Could you check a few things on this model? Use its own coordinates, in mm. A direction names the side the tool comes from. Round coordinates to 2 decimals unless told otherwise and drop trailing zeros. Order: outer loops, then holes, each group sorted by start corner. A loop starts at its lowest first (then second) coordinate and runs counter-clockwise, first axis right, second up. Notation, with made-up numbers: (40.25, 11.5) - (69.25, 11.5) arc R32 ccw to (69.25, 42.5) - close; hole circle Ø2 at (-30, 18.25). An arc over 180 degrees is marked (long way). Use one line per item in the form item = value.
from build123d import *

# Parameters (mm, degrees)
F0_R     = 100
F1_DEPTH = 3
F2_R     = 80
F3_DEPTH = 15
F4_R     = 77
F5_DEPTH = 18.001
F6_R     = 2.1
F6_R_2   = 2
F6_R_3   = 1
F7_DEPTH = 3.001


with BuildPart() as f1:
    # F0 (on Front) → F1 (new body)
    with BuildSketch(Plane.XZ):
        Circle(F0_R)
    extrude(amount=F1_DEPTH)

    # F2 (on face) → F3 (join)
    with BuildSketch(Plane.XZ.offset(3)):
        Circle(F2_R)
    extrude(amount=F3_DEPTH)

    # F4 (on face) → F5 (cut, through all)
    with BuildSketch(Plane.XZ.offset(18)):
        Circle(F4_R)
    extrude(amount=-F5_DEPTH, mode=Mode.SUBTRACT)

    # F6 (on face) → F7 (cut, through all)
    with BuildSketch(Plane.XZ.offset(3)):
        with Locations((80.622577, 40)):
            Circle(F6_R)
        with Locations((-80.622577, 40)):
            Circle(F6_R_2)
        with Locations((-80.622577, -40)):
            Circle(F6_R_2)
        with Locations((80.622577, -40)):
            Circle(F6_R_2)
        with Locations((80.770344, 0)):
            Circle(F6_R_3)
    extrude(amount=-F7_DEPTH, mode=Mode.SUBTRACT)


solid = f1.part
Item 1: Imagine slicing it at A-A on x = 0. Please give me the cut outline in (y, z).
Found:
outline = (-18, -80) - (-3, -80) - (-3, -100) - (0, -100) - (0, -77) - (-18, -77) - close; (-18, 77) - (0, 77) - (0, 100) - (-3, 100) - (-3, 80) - (-18, 80) - close
Item 2: Will these pins go through, and if not, where does the flat tip stop? P1, Ø3, axis at x = 14.5, y = -11, coming from the +Z side; P2, Ø1.5, axis at x = 26, y = -15.5, coming from the -Z side; P3, Ø4.5, axis at x = -80.62, z = 40, coming from the -Y side.
Found:
P1 = 78.94
P2 = -75.91
P3 = -3
Item 3: Imagine slicing it at D-D on x = -86. Please give me the cut outline in (y, z).
Found:
outline = (-3, -51.03) - (0, -51.03) - (0, 51.03) - (-3, 51.03) - close
Item 4: Imagine slicing it at C-C on y = -10. Please give me the cut outline in (x, z), plus the area to 3 significant figures.
Found:
outline = circle Ø160 at (0, 0); hole circle Ø154 at (0, 0)
area = 1,480 mm2
Item 5: I need wall thicknesses on L1, parallel to X at y = -11.75, z = -2 (3 decimals); L2, parallel to Z at x = 36, y = -2. Which ranges of each line are inside material? Lowest first, please.
Found:
L1 = -79.975 to -76.974, 76.974 to 79.975
L2 = -93.3 to -68.07, 68.07 to 93.3
Item 6: For faces 1 (the face through (-17.34, -10.4, -78.1)), 2 (the face through (-42, -18, 66)), which set-ups out of +Z, -Z, +X, -X, +Y, -Y let a thin tool reach every point of the face, with its end or its side?
Found:
face_1 = -Y
face_2 = +Z, -Z, +X, -X, -Y
Item 7: Imagine slicing it at B-B on z = 19.5. Please give me the cut outline in (x, y), plus the area to 3 significant figures.
Found:
outline = (-98.08, -3) - (-77.59, -3) - (-77.59, -18) - (-74.49, -18) - (-74.49, 0) - (-98.08, 0) - close; (74.49, -18) - (77.59, -18) - (77.59, -3) - (98.08, -3) - (98.08, 0) - (74.49, 0) - close
area = 234 mm2
